Geometry check sheet. Reference: the model listing, model coordinates, mm. A direction names the side the tool comes from. Round coordinates to 2 decimals unless told otherwise and drop trailing zeros. Order: outer loops, then holes, each group sorted by start corner. A loop starts at its lowest first (then second) coordinate and runs counter-clockwise, first axis right, second up. Notation, with made-up numbers: (89.5, 78.25) - (138.5, 78.25) arc R22 ccw to (138.5, 110.25) - close; hole circle Ø11 at (-30, -31.75). An arc over 180 degrees is marked (long way). Write each question's results on one line, items separated by ' | '.
```python
from build123d import *

# Parameters (mm, degrees)
SKETCH1_W                     = 50
SKETCH1_H                     = 2
BASE_FLANGE1_DEPTH            = 6.35
EDGE_FLANGE2_DEPTH            = 50
CBORE_FOR_M3_SHCS1_AT_2_COUNT = 2
CBORE_FOR_M3_SHCS1_AT_2_PITCH = 30
EDGE_FLANGE3_DEPTH            = 74.6
CUT_EXTRUDE2_START            = 10
SKETCH23_R                    = 3.25
CUT_EXTRUDE2_DEPTH            = 10


# Sheet-metal steps are written as plain solids
with BuildPart() as part:
    # Sketch1 → Base-Flange1 (new body)
    with BuildSketch(Plane(origin=(0, 0, 0), x_dir=(1, 0, 0), z_dir=(0, 1, 0))):
        Rectangle(SKETCH1_W, SKETCH1_H)
    extrude(amount=-BASE_FLANGE1_DEPTH)

    # Edge-Flange2 section (across the edge) → Edge-Flange2 (add)
    with BuildSketch(Plane(origin=(-25, 0, 20.05), x_dir=(0, 0, -1), z_dir=(1, 0, 0))):
        with BuildLine():
            Line((-6.35, 19.05), (-6.35, 93.65))
            Line((-6.35, 93.65), (0, 93.65))
            Line((0, 93.65), (0, 19.05))
            ThreePointArc((0, 19.05), (5.579615818, 5.579615818), (19.05, 0))
            Line((19.05, 0), (19.05, -6.35))
            ThreePointArc((19.05, -6.35), (1.089487758, 1.089487758), (-6.35, 19.05))
        make_face()
    extrude(amount=EDGE_FLANGE2_DEPTH)

    # Sketch19 → CBORE for M3 SHCS1 (revolve, cut)
    with BuildSketch(Plane(origin=(-15, 0, 4), x_dir=(0, 0, 1), z_dir=(1, 0, 0))):
        Polygon((0, 0), (0, 6.35), (1.8, 6.35), (1.8, 3), (3.25, 3), (3.25, 0), align=None)
    cbore_for_m3_shcs1 = revolve(axis=Axis((-15, 6.35, 4), (0, -1, 0)), mode=Mode.SUBTRACT)

    # CBORE for M3 SHCS1 at 2: CBORE for M3 SHCS1 ×2
    with Locations(*[(i * CBORE_FOR_M3_SHCS1_AT_2_PITCH, 0, 0) for i in range(1, CBORE_FOR_M3_SHCS1_AT_2_COUNT)]):
        add(cbore_for_m3_shcs1, mode=Mode.SUBTRACT)

    # Edge-Flange3 section (across the edge) → Edge-Flange3 (add)
    with BuildSketch(Plane(origin=(44.05, 19.05, 26.4), x_dir=(-1, 0, 0), z_dir=(0, 1, 0))):
        with BuildLine():
            Line((-6.35, 19.05), (-6.35, 93.65))
            Line((-6.35, 93.65), (0, 93.65))
            Line((0, 93.65), (0, 19.05))
            ThreePointArc((0, 19.05), (5.579615818, 5.579615818), (19.05, 0))
            Line((19.05, 0), (19.05, -6.35))
            ThreePointArc((19.05, -6.35), (1.089487758, 1.089487758), (-6.35, 19.05))
        make_face()
    extrude(amount=EDGE_FLANGE3_DEPTH)

    # Sketch23 → Cut-Extrude2 (cut)
    with BuildSketch(Plane(origin=(0, 0, 0), x_dir=(1, 0, 0), z_dir=(0, 1, 0)).offset(CUT_EXTRUDE2_START)):
        with Locations(Location((15, -4, 0), (0, 0, 270))):
            Circle(SKETCH23_R)
        with Locations(Location((-15, -4, 0), (0, 0, 270))):
            Circle(SKETCH23_R)
    extrude(amount=-CUT_EXTRUDE2_DEPTH, mode=Mode.SUBTRACT)


solid = part.part
```
(1) Section check D-D (z = 23). Record the cut outline in (x, y), then the cut area to 3 significant figures.
Answers follow:
outline: (-25, 6.36) - (25, 6.36) - (25, 19.05) - (36.88, 19.05) - (36.88, 93.65) - (-25, 93.65) - close | area: 5,250 mm²
(2) Depth check by flat-ended pin: pin 1 Ø1.5 at (x, y) = (7.5, 8) entering from +Z; pin 2 Ø7.5 at (x, z) = (-15, 4) entering from +Y; pin 3 Ø5 at (x, z) = (-13.5, 4.5) entering from +Y; pin 4 Ø3 at (x, z) = (-15, 4) entering from +Y. Enter the tip coordinate at first touch or a pass-through.
Answers follow:
pin 1: z = 24.22 | pin 2: y = 1.24 | pin 3: y = 0.97 | pin 4: through
(3) Access from +Z, -Z, +X, -X, +Y, -Y to the whole of each face (thin tool, end or side, straight path). Record for faces 4 (the face through (44.2, 19.05, 66.6)), 5 (the face through (0, 57, 20.05)), 6 (the face through (14.92, -4.64, 2.2)), 7 (the face through (16.4, -3, 2.6)), 8 (the face through (44.05, 56, 83)).
Answers follow:
face 4: +Z, -Z, +X, -Y | face 5: -Z, +X, -X, +Y | face 6: +Y, -Y | face 7: +Y | face 8: +Z, -X, +Y, -Y
(4) Section check A-A (z = 4). Record the cut outline in (x, y).
Answers follow:
outline: (-25, -6.17) - (-16.8, -6.17) - (-16.8, -3) - (-18.25, -3) - (-18.25, 0.24) - (-25, 0.24) - close; (-13.2, -6.17) - (13.2, -6.17) - (13.2, -3) - (11.75, -3) - (11.75, 0.24) - (-11.75, 0.24) - (-11.75, -3) - (-13.2, -3) - close; (16.8, -6.17) - (25, -6.17) - (25, 0.24) - (18.25, 0.24) - (18.25, -3) - (16.8, -3) - close
(5) Section check C-C (x = 21). Record the cut outline in (y, z).
Answers follow:
outline: (-6.35, -1) - (0, -1) - (0, 1) arc R19.05 cw to (19.05, 20.05) - (93.65, 20.05) - (93.65, 26.4) - (19.05, 26.4) arc R25.4 ccw to (-6.35, 1) - close
(6) Draft check along Z on faces 1 (the face through (42.76, 55.83, 27.29)), 2 (the face through (-13.6, -3, 2.6)), 3 (the face through (25, 5, 15)). Enter one of: released by +Z, released by -Z, zero draft, split by the parting line, or undercut.
Answers follow:
face 1: released by -Z | face 2: undercut | face 3: zero draft
(7) Material ranges on line 1 (X direction, y = -4, z = 4); line 2 (X direction, y = 0, z = 4); line 3 (X direction, y = 79.5, z = 97), recorded low to high.
Answers follow:
line 1: -25 to -16.8, -13.2 to 13.2, 16.8 to 25 | line 2: -25 to -18.25, -11.75 to 11.75, 18.25 to 25 | line 3: 44.05 to 50.4
(8) Section check B-B (y = 20.5). Record the cut outline in (x, z), then the cut area to 3 significant figures.
Answers follow:
outline: (-25, 20.05) - (25, 20.05) arc R25.4 ccw to (50.4, 45.45) - (50.4, 120.05) - (44.05, 120.05) - (44.05, 45.45) arc R19.05 cw to (25, 26.4) - (-25, 26.4) - close | area: 1,010 mm²
